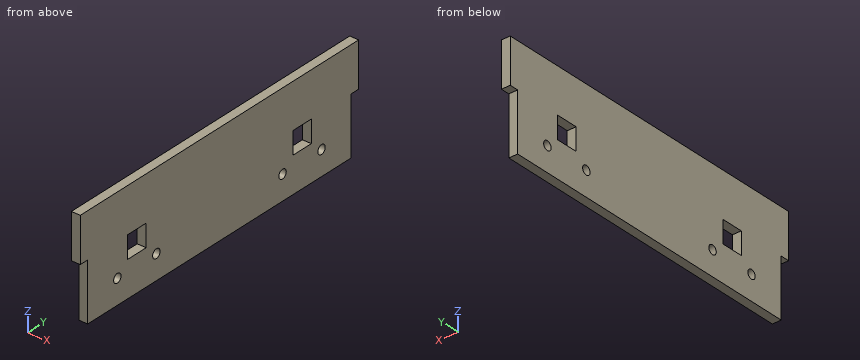
```python
from build123d import *

# Parameters (mm, degrees)
SKETCH_W        = 150
SKETCH_H        = 46
PAD_DEPTH       = 4
SKETCH001_W     = 4
SKETCH001_H     = 26
POCKET_DEPTH    = 5
SKETCH002_R     = 2
SKETCH002_W     = 10
SKETCH002_H     = 10
POCKET001_DEPTH = 5


with BuildPart() as part:
    # Sketch → Pad (new body)
    with BuildSketch(Plane.YZ):
        with Locations((75, 23)):
            Rectangle(SKETCH_W, SKETCH_H)
    extrude(amount=PAD_DEPTH)

    # Sketch001 (on Face6 of Pad) → Pocket (cut)
    with BuildSketch(Plane.YZ.offset(4)):
        with Locations((2, 13)):
            Rectangle(SKETCH001_W, SKETCH001_H)
        with Locations((148, 13)):
            Rectangle(SKETCH001_W, SKETCH001_H)
    extrude(amount=-POCKET_DEPTH, mode=Mode.SUBTRACT)

    # Sketch002 (on Face4 of Pocket) → Pocket001 (cut)
    with BuildSketch(Plane.YZ.offset(4)):
        with Locations((20, 11)):
            Circle(SKETCH002_R)
        with Locations((41, 11)):
            Circle(SKETCH002_R)
        with Locations((109, 11)):
            Circle(SKETCH002_R)
        with Locations((130, 11)):
            Circle(SKETCH002_R)
        with Locations((30.5, 21)):
            Rectangle(SKETCH002_W, SKETCH002_H)
        with Locations((119.5, 21)):
            Rectangle(SKETCH002_W, SKETCH002_H)
    extrude(amount=-POCKET001_DEPTH, mode=Mode.SUBTRACT)


solid = part.part
```
Input: part model. Units: mm. Frame: model coordinates. Coordinates: 2 decimals unless noted, no trailing zeros. Loops run counter-clockwise (first coordinate to the right, second up) from the corner with the lowest first, then second, coordinate; pieces in that order, holes last. Notation, with made-up numbers: (64.5, -7.5) - (98.5, -7.5) arc R8 ccw to (98.5, 0.5) - close; hole circle Ø5 at (13.25, -30.5). An arc over 180 degrees is marked (long way). Answer in a Markdown table with one row per item.
(1) Cut plane C-C on x = 0.6. Output: boundary loops of the cut face in (y, z).
Model answer:
| item | result |
|---|---|
| outline | (0, 26) - (4, 26) - (4, 0) - (146, 0) - (146, 26) - (150, 26) - (150, 46) - (0, 46) - close; hole circle Ø4 at (20, 11); hole (25.5, 16) - (35.5, 16) - (35.5, 26) - (25.5, 26) - close; hole circle Ø4 at (41, 11); hole circle Ø4 at (109, 11); hole (114.5, 16) - (124.5, 16) - (124.5, 26) - (114.5, 26) - close; hole circle Ø4 at (130, 11) |
(2) Cut plane A-A on z = 11. Output: boundary loops of the cut face in (x, y), plus the area to 3 significant figures.
Model answer:
| item | result |
|---|---|
| outline | (0, 4) - (4, 4) - (4, 18) - (0, 18) - close; (0, 22) - (4, 22) - (4, 39) - (0, 39) - close; (0, 43) - (4, 43) - (4, 107) - (0, 107) - close; (0, 111) - (4, 111) - (4, 128) - (0, 128) - close; (0, 132) - (4, 132) - (4, 146) - (0, 146) - close |
| area | 504 mm² |
(3) Material intervals for L1, parallel to Y at x = 2.55, z = 17; L2, parallel to Z at x = 2.75, y = 20; L3, parallel to Y at x = 3.1, z = 10.5, sorted ascending. Write a range as from..to.
Model answer:
| item | result |
|---|---|
| L1 | y = 4..25.5, 35.5..114.5, 124.5..146 |
| L2 | z = 0..9, 13..46 |
| L3 | y = 4..18.06, 21.94..39.06, 42.94..107.06, 110.94..128.06, 131.94..146 |
(4) Cut plane D-D on z = 4. Output: boundary loops of the cut face in (x, y), plus the area to 3 significant figures.
Model answer:
| item | result |
|---|---|
| outline | (0, 4) - (4, 4) - (4, 146) - (0, 146) - close |
| area | 568 mm² |
(5) Pin query (flat end, axial travel): P1, Ø3, axis at y = 109, z = 11, coming from the +X side; P2, Ø1.2, axis at x = 2, z = 19, coming from the -Y side; P3, Ø2, axis at x = 2.5, z = 20.5, coming from the +Y side. Return the tip coordinate at first contact, or that it passes through.
Model answer:
| item | result |
|---|---|
| P1 | passes through |
| P2 | stops at y = 4 |
| P3 | stops at y = 146 |
(6) Cut plane B-B on y = 41. Output: boundary loops of the cut face in (x, z).
Model answer:
| item | result |
|---|---|
| outline | (0, 0) - (4, 0) - (4, 9) - (0, 9) - close; (0, 13) - (4, 13) - (4, 46) - (0, 46) - close |
